from build123d import *

# Parameters (mm, degrees)
SKETCH1_R                = 24
BOSS_EXTRUDE1_DEPTH      = 42
FILLET1_R                = 3
BOSS_EXTRUDE2_DEPTH      = 18
BOSS_EXTRUDE2_DEPTH_BACK = 18
CUT_EXTRUDE2_DEPTH       = 42
CUT_EXTRUDE3_DEPTH       = 62.400856059
CUT_EXTRUDE3_DEPTH_BACK  = 62.400856059
FILLET2_R                = 6
FILLET3_R                = 8
FILLET4_R                = 3
SKETCH6_W                = 32
SKETCH6_H                = 1.990473873
SKETCH6_H_2              = 40.942974084
CUT_EXTRUDE5_DEPTH       = 40
SKETCH7_R                = 16
BOSS_EXTRUDE3_DEPTH      = 1
SKETCH8_R                = 10
CUT_EXTRUDE6_DEPTH       = 3
CHAMFER1_SIZE            = 3
SKETCH9_R                = 5
BOSS_EXTRUDE4_DEPTH      = 4
CHAMFER2_SIZE            = 1
SKETCH10_R               = 3
CUT_EXTRUDE7_DEPTH       = 71.095779947
SKETCH11_R               = 7.5
BOSS_EXTRUDE5_DEPTH      = 2
SKETCH12_R               = 21
BOSS_EXTRUDE6_DEPTH      = 1
DOME1_FACE_RADIUS        = 21
DOME1_HEIGHT             = 10
BOSS_EXTRUDE7_START      = -30
SKETCH13_R               = 5
BOSS_EXTRUDE7_DEPTH      = 30
SCALE1_SCALE             = 0.7761


# Some blends are built 0.0001 mm under size
with BuildPart() as part:
    # Sketch1 → Boss-Extrude1 (new body)
    with BuildSketch(Plane(origin=(0, 0, 0), x_dir=(1, 0, 0), z_dir=(0, 1, 0))):
        with Locations(Location((0, 0, 0), (0, 0, 90))):
            Circle(SKETCH1_R)
    extrude(amount=BOSS_EXTRUDE1_DEPTH)

    # Fillet1
    fillet1_edges = [part.edges().sort_by_distance(p)[0] for p in [
        (0, 42, 24),
    ]]
    fillet(fillet1_edges, radius=FILLET1_R)

    # Sketch2 → Boss-Extrude2 (add, two sides: drawn at the far end of the back side and taken through both)
    with BuildSketch(Plane(origin=(0, 0, 0), x_dir=(0, 0, -1), z_dir=(1, 0, 0)).offset(-BOSS_EXTRUDE2_DEPTH_BACK)):
        Polygon((-24, 39), (-33.81365361, 39), (-37.816201771, -3.269008091), (-26.156604955, -3.269008091), (15.957162651, 34.668187521), (24, 34.668187521), (24, 39), align=None)
    extrude(amount=BOSS_EXTRUDE2_DEPTH + BOSS_EXTRUDE2_DEPTH_BACK)

    # Sketch4 → Cut-Extrude2 (cut)
    with BuildSketch(Plane.XZ):
        with BuildLine():
            Line((23.002581612, -9.203628547), (22.165135271, -9.203628547))
            ThreePointArc((22.165135271, -9.203628547), (0, -24), (-22.165135271, -9.203628547))
            Line((-22.165135271, -9.203628547), (-22.165135271, -25.095490922))
            Line((-22.165135271, -25.095490922), (23.002581612, -25.095490922))
            Line((23.002581612, -25.095490922), (23.002581612, -9.203628547))
        make_face()
    extrude(amount=-CUT_EXTRUDE2_DEPTH, mode=Mode.SUBTRACT)

    # Sketch5 → Cut-Extrude3 (cut, two sides: drawn at the far end of the back side and taken through both)
    with BuildSketch(Plane(origin=(0, 0, 0), x_dir=(0, 0, -1), z_dir=(1, 0, 0)).offset(-CUT_EXTRUDE3_DEPTH_BACK)):
        Polygon((-26.156604955, -3.269008091), (14.621999629, 33.5), (25.781931598, 33.5), (25.781931598, -3.269008091), align=None)
    extrude(amount=CUT_EXTRUDE3_DEPTH + CUT_EXTRUDE3_DEPTH_BACK, mode=Mode.SUBTRACT)

    # Fillet2
    fillet2_edges = [part.edges().sort_by_distance(p)[0] for p in [
        (0, -3.269008091, 37.816201771),
    ]]
    fillet(fillet2_edges, radius=FILLET2_R)

    # Fillet3
    fillet3_edges = [part.edges().sort_by_distance(p)[0] for p in [
        (0, -3.269008091, 26.156604955),
    ]]
    fillet(fillet3_edges, radius=FILLET3_R)

    # Fillet4
    # the kernel refuses this fillet: 3 mm, written as the material it takes off along each edge
    with BuildSketch(Plane(origin=(18, 39, 41.31365361), x_dir=(-1, 0, 0), z_dir=(0, 0, -1))) as fillet4_piece_1_section:
        with BuildLine():
            CenterArc((FILLET4_R, -FILLET4_R), FILLET4_R, 90, 90)
            Line((0, -FILLET4_R), (0, 0))
            Line((0, 0), (FILLET4_R, 0))
        make_face()
    fillet4_piece_1 = extrude(amount=32.939145744, mode=Mode.PRIVATE)
    fillet4_piece_1 = fillet4_piece_1 - Plane(origin=(0, 38.317129028, 0), x_dir=(0, 0, -1), z_dir=(0, -1, 0)) * Cylinder(24, 78, mode=Mode.PRIVATE)
    add(fillet4_piece_1, mode=Mode.SUBTRACT)
    with BuildSketch(Plane(origin=(-18, 39, 8.374507866), x_dir=(0, -1, 0), z_dir=(0, 0, 1))) as fillet4_piece_2_section:
        with BuildLine():
            CenterArc((FILLET4_R, FILLET4_R), FILLET4_R, 180, 90)
            Line((0, FILLET4_R), (0, 0))
            Line((0, 0), (FILLET4_R, 0))
        make_face()
    fillet4_piece_2 = extrude(amount=32.939145744, mode=Mode.PRIVATE)
    fillet4_piece_2 = fillet4_piece_2 - Plane(origin=(0, 38.317126887, 0), x_dir=(0, 0, -1), z_dir=(0, -1, 0)) * Cylinder(24, 78, mode=Mode.PRIVATE)
    add(fillet4_piece_2, mode=Mode.SUBTRACT)

    # Sketch6 → Cut-Extrude5 (cut)
    with BuildSketch(Plane.XZ.offset(3.269008091)):
        with BuildLine():
            ThreePointArc((16, 15.099668871), (0, 22), (-16, 15.099668871))
            Line((-16, 15.099668871), (-16, 2.278234246))
            Line((-16, 2.278234246), (16, 2.278234246))
            Line((16, 2.278234246), (16, 15.099668871))
        make_face()
        with BuildLine():
            Line((-16, 2.278234246), (-16, 15.099668871))
            ThreePointArc((-16, 15.099668871), (-8.124038405, -20.4450483), (22, 0))
            ThreePointArc((22, 0), (20.4450483, 8.124038405), (16, 15.099668871))
            Line((16, 15.099668871), (16, 2.278234246))
            Line((16, 2.278234246), (-16, 2.278234246))
        make_face()
        with Locations((0, 30.225971395)):
            Rectangle(SKETCH6_W, SKETCH6_H)
        with Locations((0, 51.692695373)):
            Rectangle(SKETCH6_W, SKETCH6_H_2)
        with BuildLine():
            Line((16, 29.230734458), (-16, 29.230734458))
            Line((-16, 29.230734458), (-16, 15.099668871))
            ThreePointArc((-16, 15.099668871), (0, 22), (16, 15.099668871))
            Line((16, 15.099668871), (16, 29.230734458))
        make_face()
    extrude(amount=-CUT_EXTRUDE5_DEPTH, mode=Mode.SUBTRACT)

    # Sketch7 → Boss-Extrude3 (add)
    with BuildSketch(Plane.XZ.offset(-36.730991909)):
        with Locations(Location((0, 0, 0), (0, 0, 270))):
            Circle(SKETCH7_R)
    extrude(amount=BOSS_EXTRUDE3_DEPTH)

    # Sketch8 → Cut-Extrude6 (cut)
    with BuildSketch(Plane.XZ.offset(-35.730991909)):
        with Locations(Location((0, 0, 0), (0, 0, 270))):
            Circle(SKETCH8_R)
    extrude(amount=-CUT_EXTRUDE6_DEPTH, mode=Mode.SUBTRACT)

    # Chamfer1
    chamfer1_edges = [part.edges().sort_by_distance(p)[0] for p in [
        (0, 38.730991909, 10),
    ]]
    chamfer(chamfer1_edges, length=CHAMFER1_SIZE - 0.0001)  # a hair under: the kernel refuses the full size

    # Sketch9 → Boss-Extrude4 (add)
    with BuildSketch(Plane.XZ.offset(-38.730991909)):
        with Locations(Location((0, 0, 0), (0, 0, 270))):
            Circle(SKETCH9_R)
    extrude(amount=BOSS_EXTRUDE4_DEPTH)

    # Chamfer2
    chamfer2_edges = [part.edges().sort_by_distance(p)[0] for p in [
        (0, 34.730991909, 5),
    ]]
    chamfer(chamfer2_edges, length=CHAMFER2_SIZE)

    # Sketch10 → Cut-Extrude7 (cut, through all)
    with BuildSketch(Plane(origin=(18, 0, 0), x_dir=(0, 0, -1), z_dir=(1, 0, 0))):
        with Locations((-29.763213514, 2.730991909)):
            Circle(SKETCH10_R)
    extrude(amount=-CUT_EXTRUDE7_DEPTH, mode=Mode.SUBTRACT)

    # Sketch11 → Boss-Extrude5 (add)
    with BuildSketch(Plane(origin=(0, 42, 0), x_dir=(1, 0, 0), z_dir=(0, 1, 0))):
        with Locations(Location((0, 0, 0), (0, 0, 270))):
            Circle(SKETCH11_R)
    extrude(amount=BOSS_EXTRUDE5_DEPTH)

    # Sketch12 → Boss-Extrude6 (add)
    with BuildSketch(Plane(origin=(0, 44, 0), x_dir=(1, 0, 0), z_dir=(0, 1, 0))):
        with Locations(Location((0, 0, 0), (0, 0, 270))):
            Circle(SKETCH12_R)
    extrude(amount=BOSS_EXTRUDE6_DEPTH)

    # Dome1: a dome of height H over a round flat face of radius A is a cap of a sphere of radius (A * A + H * H) / (2 * H)
    dome1_r = (DOME1_FACE_RADIUS * DOME1_FACE_RADIUS + DOME1_HEIGHT * DOME1_HEIGHT) / (2 * DOME1_HEIGHT)
    dome1_base = Plane((0, 45, 0), z_dir=(0, 1, 0))
    with Locations(dome1_base.offset(DOME1_HEIGHT - dome1_r)):
        dome1_ball = Sphere(dome1_r, mode=Mode.PRIVATE)
    add(split(dome1_ball, bisect_by=dome1_base, keep=Keep.TOP, mode=Mode.PRIVATE))

    # Sketch13 → Boss-Extrude7 (add)
    with BuildSketch(Plane.XZ.offset(-34.730991909).offset(BOSS_EXTRUDE7_START)):
        with Locations(Location((0, 0, 0), (0, 0, 270))):
            Circle(SKETCH13_R)
    extrude(amount=BOSS_EXTRUDE7_DEPTH)


with BuildPart() as part_1:
    # Scale1: scaled about (-4.3e-08, 39.220241586, 4.118564184)
    add(part.part.scale(SCALE1_SCALE).moved(Location((-1e-08, 8.781412091, 0.922146521))))


solid = part_1.part
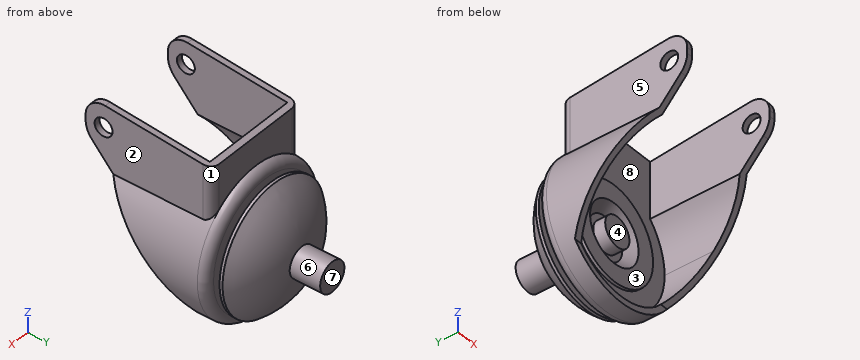
Check sheet for the modelled part. Datum: model origin and axes. Units: mm. Face numbers are marked on the shaded views. A direction names the side the tool comes from. Coordinates: 2 decimals unless noted, no trailing zeros. Write each loop counter-clockwise with the first axis right and the second up, starting at its lowest first coordinate (ties: lowest second). Pieces come first, ordered by that corner, then holes.
Item 1: Access from +Z, -Z, +X, -X, +Y, -Y to the whole of each face (thin tool, end or side, straight path). Record for the marked faces 1, 2, 3, 4 and 5.
Numbers:
face 1: +Z, +X, +Y
face 2: +Z, +X, +Y, -Y
face 3: -Y
face 4: +Z, -Y
face 5: +Z, -X, +Y, -Y
Item 2: Cross-section at B-B on y = 22. Record the boundary of the cut face in (x, z), then the cut area to 3 significant figures.
Numbers:
outline: (-18.41, 3.75) - (-16.84, 3.75) arc R17.07 cw to (-12.42, 12.64) - (-12.42, 28.78) - (-13.97, 28.78) - (-13.97, 13.24) arc R18.63 ccw to start; (12.42, 12.64) arc R17.07 cw to (16.84, 3.75) - (18.41, 3.75) arc R18.63 ccw to (13.97, 13.24) - (13.97, 28.78) - (12.42, 28.78) - close
area: 81.3 mm2
Item 3: Depth check by flat-ended pin: pin 1 Ø8 at (y, z) = (24.5, 7) entering from -X; pin 2 Ø1 at (x, z) = (11, 21) entering from -Y; pin 3 Ø3 at (x, y) = (6.5, 44.5) entering from +Z; pin 4 Ø4 at (y, z) = (10.9, 24.02) entering from +X. Enter the tip coordinate at first touch or a pass-through.
Numbers:
pin 1: stops at x = -18.51
pin 2: stops at y = 37.29
pin 3: stops at z = 16.36
pin 4: passes through
Item 4: Cross-section at A-A on z = 22.5. Record the boundary of the cut face in (x, y).
Numbers:
outline: (-13.97, 6.34) - (-12.42, 6.34) - (-12.42, 9.14) - (-13.97, 9.14) - close; (-13.97, 12.66) - (-12.42, 12.66) - (-12.42, 37.29) - (12.42, 37.29) - (12.42, 12.66) - (13.97, 12.66) - (13.97, 36.72) arc R2.33 ccw to (11.64, 39.05) - (-11.64, 39.05) arc R2.33 ccw to (-13.97, 36.72) - close; (12.42, 6.34) - (13.97, 6.34) - (13.97, 9.14) - (12.42, 9.14) - close
Item 5: Mould release check, pull along Z, two halves, no side actions. Record for the marked faces 6, 7 and 8: released by +Z, released by -Z, zero draft, split by the parting line, or undercut.
Numbers:
face 6: split by the parting line
face 7: zero draft
face 8: undercut
Item 6: Cross-section at C-C on y = 49.5. Record the boundary of the cut face in (x, z).
Numbers:
outline: circle Ø17.74 at (0, 0.92)
Item 7: Scan lines: probe 1 along Z at (x, y) = (0, 36); probe 2 along X at (y, z) = (34, 15); probe 3 along Y at (x, z) = (-3.5, -14). Record each from-to range of solid material in increasing order.
Numbers:
probe 1: z = -17.7 to -16.15, -2.96 to 4.8
probe 2: x = -13.97 to -12.42, 12.42 to 13.97
probe 3: y = 37.29 to 41.38, 42.93 to 44.82
